The drawing under review shows one solid part. Ordinate dimensions are in mm from its lowest x, y, z. A direction names the side the tool comes from. Round coordinates to 2 decimals unless told otherwise and drop trailing zeros. Write each loop counter-clockwise with the first axis right and the second up, starting at its lowest first coordinate (ties: lowest second). Pieces come first, ordered by that corner, then holes. Notation, with made-up numbers: (-31, -4) -> (-2, -4) arc R11 cw to (-2, 7) -> close; hole circle Ø8 at (73.5, 52.25). An arc over 180 degrees is marked (long way). Use CSV: the item, a comma, the result in double quotes. Start each with the question number.
1) Take a section at B-B, the plane z = 1.25. Give the boundary of the cut face in (x, y) (3 decimals), then the cut area to 3 significant figures.
2) Take a section at A-A, the plane x = 15. Give the boundary of the cut face in (y, z) (3 decimals).
3) Take a section at D-D, the plane z = 3.5. Give the boundary of the cut face in (x, y) (3 decimals).
4) Take a section at C-C, the plane y = 1.5. Give the boundary of the cut face in (x, z).
5) Wall thickness on probe 1 along Y at (x, z) = (40, 9) (3 decimals); probe 2 along Y at (x, z) = (40, 4) (3 decimals); probe 3 along X at (y, z) = (7.75, 9.25): over which ranges is each line inside the solid? List them lowest first. Write a range as [from, to].
6) Mouldability with a two-part tool opening along Y and no side actions: class the marked faces 4, 5 and 6 as released by +Y, released by -Y, zero draft, split by the parting line, or undercut.
7) Machinability: for the marked faces 1, 2 and 3, which of the approach directions +Z, -Z, +X, -X, +Y, -Y give a long, thin tool a straight path to every point of the face, cutting with its end or side? Answer none if there is none.
8) For pin 1 Ø1.5 at (x, z) = (13.5, 3.5) entering from -Y; pin 2 Ø1.5 at (x, z) = (28, 2) entering from +Y; pin 3 Ø1.8 at (x, y) = (15.5, 6.5) entering from -Z; pin 4 Ø1.5 at (x, z) = (24, 3) entering from -Y, all flat-tipped, find the tip position at first contact; note any pin that passes through.
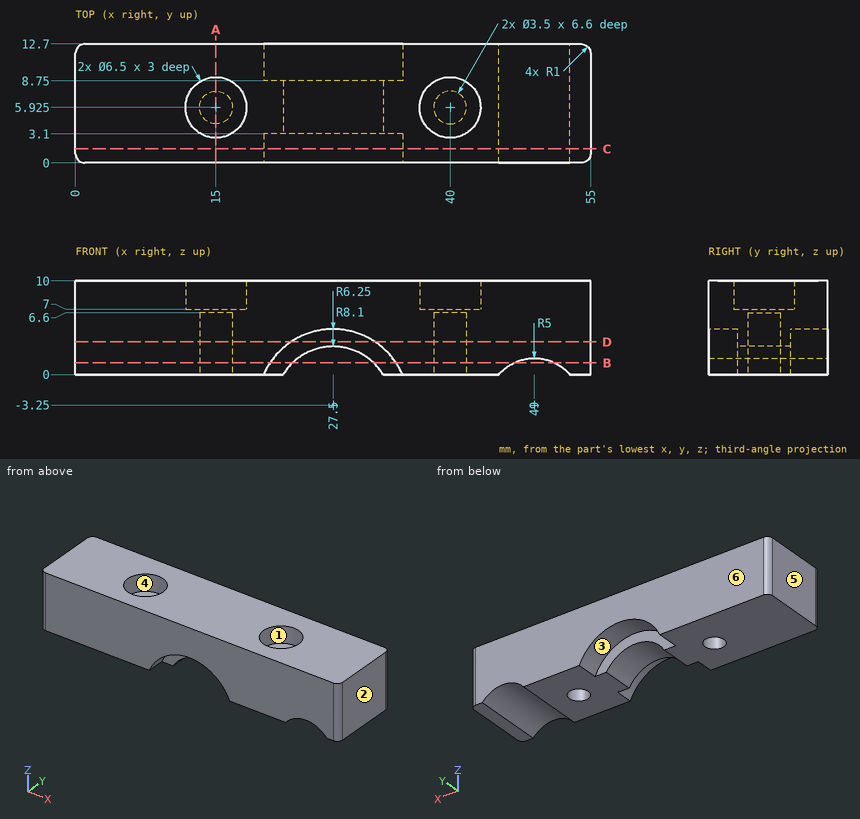
Values found:
1,outline,"(0, 1) arc R1 ccw to (1, 0) -> (20.765, 0) -> (20.765, 3.1) -> (23.163, 3.1) -> (23.163, 8.75) -> (20.765, 8.75) -> (20.765, 12.7) -> (1, 12.7) arc R1 ccw to (0, 11.7) -> close; (31.837, 3.1) -> (34.235, 3.1) -> (34.235, 0) -> (46.821, 0) -> (46.821, 12.7) -> (34.235, 12.7) -> (34.235, 8.75) -> (31.837, 8.75) -> close; (51.179, 0) -> (54, 0) arc R1 ccw to (55, 1) -> (55, 11.7) arc R1 ccw to (54, 12.7) -> (51.179, 12.7) -> close; hole circle Ø3.5 at (15, 5.925); hole circle Ø3.5 at (40, 5.925)"
1,area,"479 mm²"
2,outline,"(0, 0) -> (4.175, 0) -> (4.175, 6.6) -> (7.675, 6.6) -> (7.675, 0) -> (12.7, 0) -> (12.7, 10) -> (9.175, 10) -> (9.175, 7) -> (2.675, 7) -> (2.675, 10) -> (0, 10) -> close"
3,outline,"(0, 1) arc R1 ccw to (1, 0) -> (23.023, 0) -> (23.023, 3.1) -> (31.977, 3.1) -> (31.977, 0) -> (54, 0) arc R1 ccw to (55, 1) -> (55, 11.7) arc R1 ccw to (54, 12.7) -> (31.977, 12.7) -> (31.977, 8.75) -> (23.023, 8.75) -> (23.023, 12.7) -> (1, 12.7) arc R1 ccw to (0, 11.7) -> close; hole circle Ø3.5 at (15, 5.925); hole circle Ø3.5 at (40, 5.925)"
4,outline,"(0, 0) -> (20.08, 0) arc R8.1 cw to (34.92, 0) -> (45.2, 0) arc R5 cw to (52.8, 0) -> (55, 0) -> (55, 10) -> (0, 10) -> close"
5,probe 1,"[0, 2.675], [9.175, 12.7]"
5,probe 2,"[0, 4.175], [7.675, 12.7]"
5,probe 3,"[0, 12.31], [17.69, 37.31], [42.69, 55]"
6,face 4,"undercut"
6,face 5,"zero draft"
6,face 6,"released by +Y"
7,face 1,"+Z"
7,face 2,"+Z, -Z, +X, +Y, -Y"
7,face 3,"-Z, +Y"
8,pin 1,"y = 0"
8,pin 2,"through"
8,pin 3,"z = 6.6"
8,pin 4,"y = 3.1"
